Source: CAD feature listing. Evaluate the final solid. Frame: model axes, mm. A direction names the side the tool comes from. Give positions to 0.01 mm unless a question says otherwise; leave off trailing zeros. Loops run counter-clockwise (first coordinate to the right, second up) from the corner with the lowest first, then second, coordinate; pieces in that order, holes last. Notation, with made-up numbers: M 44,79.25 L 61,79.25 A14 cw 61,86.25 Z; hole C -28,11.5 d7. An arc over 180 degrees is marked long. Answer in a Markdown table with one row per item.
```python
from build123d import *

# Parameters (mm, degrees)
F1_DEPTH  = 48
F3_DEPTH  = 19
F5_DEPTH  = 19
F7_DEPTH  = 25
F9_DEPTH  = 10
F10_W     = 9.3963341787
F10_H     = 5.939177354
F11_DEPTH = 10
F12_W     = 8.2590989769
F12_H     = 6.0978346739
F13_DEPTH = 10


with BuildPart() as f1:
    # F0 (on Right) → F1 (new body)
    with BuildSketch(Plane.YZ):
        Polygon((-4.4177471522, 4.4790807286), (-2.2589041686, 4.4790807286), (-2.2589041686, 11.4790807286), (-0.2589041686, 11.4790807286), (-0.2589041686, 4.4790807286), (1.774286502, 4.4790807286), (1.774286502, 20.2315860614), (-2.5690435432, 20.2315860614), (-2.5690435432, 27.6196174324), (1.774286502, 27.6196174324), (1.774286502, 52.6196174324), (-4.4177471522, 52.6196174324), align=None)
    extrude(amount=F1_DEPTH)

    # F2 (on face) → F3 (join)
    with BuildSketch(Plane(origin=(0, 0, 0), x_dir=(0, -1, 0), z_dir=(-1, 0, 0))):
        Polygon((2.5690435432, 27.6196174324), (4.4177471522, 27.6196174324), (4.4177471522, 52.6196174324), (-1.774286502, 52.6196174324), (-1.774286502, 27.6196174324), align=None)
    extrude(amount=F3_DEPTH)

    # F4 (on face) → F5 (join)
    with BuildSketch(Plane.YZ.offset(48)):
        Polygon((1.774286502, 52.6196174324), (-4.4177471522, 52.6196174324), (-4.4177471522, 27.6196174324), (-2.5690435432, 27.6196174324), (1.774286502, 27.6196174324), align=None)
    extrude(amount=F5_DEPTH)

    # F6 (on face) → F7 (cut)
    with BuildSketch(Plane(origin=(0, 1.774286502, 0), x_dir=(-1, 0, 0), z_dir=(0, 1, 0))):
        with BuildLine():
            ThreePointArc((-61.5190799241, 52.6196174324), (-58.7365943454, 45.9021030111), (-52.0190799241, 43.1196174324))
            ThreePointArc((-52.0190799241, 43.1196174324), (-45.3015655028, 45.9021030111), (-42.5190799241, 52.6196174324))
            Line((-42.5190799241, 52.6196174324), (-61.5190799241, 52.6196174324))
        make_face()
        with BuildLine():
            ThreePointArc((-8.0190799241, 52.6196174324), (-5.2365943454, 45.9021030111), (1.4809200759, 43.1196174324))
            ThreePointArc((1.4809200759, 43.1196174324), (8.1984344972, 45.9021030111), (10.9809200759, 52.6196174324))
            Line((10.9809200759, 52.6196174324), (-8.0190799241, 52.6196174324))
        make_face()
        with BuildLine():
            ThreePointArc((-42.5190799241, 52.6196174324), (-45.3015655028, 45.9021030111), (-52.0190799241, 43.1196174324))
            Line((-52.0190799241, 43.1196174324), (1.4809200759, 43.1196174324))
            ThreePointArc((1.4809200759, 43.1196174324), (-5.2365943454, 45.9021030111), (-8.0190799241, 52.6196174324))
            Line((-8.0190799241, 52.6196174324), (-42.5190799241, 52.6196174324))
        make_face()
    extrude(amount=-F7_DEPTH, mode=Mode.SUBTRACT)

    # F8 (on face) → F9 (join)
    with BuildSketch(Plane.XZ.offset(4.4177471522)):
        Polygon((0, 36.6360321641), (0, 43.1196174324), (-1.4809200759, 43.1196174324), (-9.3963341787, 43.1196174324), (-9.3963341787, 36.6360321641), align=None)
        Polygon((52.0190799241, 43.1196174324), (49.577344209, 43.1196174324), (49.577344209, 34.7543694079), (57.8364431858, 34.7543694079), (57.8364431858, 43.1196174324), align=None)
    extrude(amount=F9_DEPTH)

    # F10 (on face) → F11 (join)
    with BuildSketch(Plane.XY.offset(43.1196174324)):
        with Locations((-4.6981670894, -11.4481584752)):
            Rectangle(F10_W, F10_H)
    extrude(amount=F11_DEPTH)

    # F12 (on face) → F13 (join)
    with BuildSketch(Plane.XY.offset(43.1196174324)):
        with Locations((53.7068936974, -11.3688298153)):
            Rectangle(F12_W, F12_H)
    extrude(amount=F13_DEPTH)


solid = f1.part
```
Q1. Mould query, pull axis X, two halves, no side actions, for faces 1 (the flat face through (64, -1, 52.62)), 2 (the flat face through (57.836, -11, 44)), 3 (the flat face through (-9.396, -11, 43)), 4 (the flat face through (49.577, -11, 44)). Classes: +X half, -X half, draft (parallel to the pull), parting line (faces both ways), or undercut.
Values follow:
| item | result |
|---|---|
| face 1 | draft |
| face 2 | +X half |
| face 3 | -X half |
| face 4 | undercut |
Q2. Section query A-A (y = -6). Output: boundary loops of the cut face in (x, z).
Values follow:
| item | result |
|---|---|
| outline | M -9.4,36.64 L 0,36.64 L 0,43.12 L -9.4,43.12 Z; M 49.58,34.75 L 57.84,34.75 L 57.84,43.12 L 49.58,43.12 Z |
Q3. Ray query, probe 1 along X at (y, z) = (-12.25, 43); probe 2 along Y at (x, z) = (32.5, 21.5); probe 3 along Y at (x, z) = (6.5, 7). Return the intervals inside material, ascending. Write a range as from..to.
Values follow:
| item | result |
|---|---|
| probe 1 | -9.4..0, 49.58..57.84 |
| probe 2 | -4.42..-2.57 |
| probe 3 | -4.42..-2.26, -0.26..1.77 |
Q4. Contact query for flat-ended pins moving along their axis: pin 1 Ø1 at (y, z) = (-4.5, 17) entering from +X; pin 2 Ø4 at (y, z) = (-7, 41) entering from +X; pin 3 Ø3 at (y, z) = (-9.5, 44) entering from -X; pin 4 Ø9 at (x, z) = (54, 47) entering from +Y. Output: stop coordinate, or through.
Values follow:
| item | result |
|---|---|
| pin 1 | x = 48 |
| pin 2 | x = 57.84 |
| pin 3 | x = -9.4 |
| pin 4 | y = 1.77 |
Q5. Reachability of faces 5 (the flat face through (24, 0, 20.232)), 6 (the flat face through (24, -1, 11.479)), 7 (the flat face through (48, -1, 14)) from +Z, -Z, +X, -X, +Y, -Y: full face, straight path, thin tool, end or side. Return the list, or none.
Values follow:
| item | result |
|---|---|
| face 5 | +X, -X, +Y |
| face 6 | -Z, +X, -X |
| face 7 | -Z, +X, +Y, -Y |
Q6. Section query D-D (y = -11.25). Output: boundary loops of the cut face in (x, z).
Values follow:
| item | result |
|---|---|
| outline | M -9.4,36.64 L 0,36.64 L 0,53.12 L -9.4,53.12 Z; M 49.58,34.75 L 57.84,34.75 L 57.84,53.12 L 49.58,53.12 Z |
Q7. Section query C-C (x = 13). Output: boundary loops of the cut face in (y, z).
Values follow:
| item | result |
|---|---|
| outline | M -4.42,4.48 L -2.26,4.48 L -2.26,11.48 L -0.26,11.48 L -0.26,4.48 L 1.77,4.48 L 1.77,20.23 L -2.57,20.23 L -2.57,27.62 L 1.77,27.62 L 1.77,43.12 L -4.42,43.12 Z |
Q8. Section query B-B (z = 44.5). Output: boundary loops of the cut face in (x, y), plus the area to 3 significant figures.
Values follow:
| item | result |
|---|---|
| outline | M -19,-4.42 L -6.41,-4.42 L -6.41,1.77 L -19,1.77 Z; M -9.4,-14.42 L 0,-14.42 L 0,-8.48 L -9.4,-8.48 Z; M 49.58,-14.42 L 57.84,-14.42 L 57.84,-8.32 L 49.58,-8.32 Z; M 56.95,-4.42 L 67,-4.42 L 67,1.77 L 56.95,1.77 Z |
| area | 246 mm^2 |
